```python
from build123d import *

# Parameters (mm, degrees)
SKETCH_1_W                         = 50
SKETCH_1_H                         = 50
SM_BASE_FLANGE_1_DEPTH             = 3
SM_EDGE_FLANGE_1_STRIP_W           = 13.4732
SM_EDGE_FLANGE_1_STRIP_H           = 3
SM_EDGE_FLANGE_1_STRIP_CUT_DEPTH   = 50
SM_EDGE_FLANGE_1_STRIP_2_W         = 13.4732
SM_EDGE_FLANGE_1_STRIP_2_H         = 3
SM_EDGE_FLANGE_1_STRIP_CUT_2_DEPTH = 50
SM_EDGE_FLANGE_1_DEPTH             = 50
SM_EDGE_FLANGE_1_BEND_DEPTH        = 50
SM_EDGE_FLANGE_2_STRIP_W           = 13.4732
SM_EDGE_FLANGE_2_STRIP_H           = 3
SM_EDGE_FLANGE_2_STRIP_CUT_DEPTH   = 50
SM_EDGE_FLANGE_2_STRIP_2_W         = 13.4732
SM_EDGE_FLANGE_2_STRIP_2_H         = 3
SM_EDGE_FLANGE_2_STRIP_CUT_2_DEPTH = 50
SM_EDGE_FLANGE_2_DEPTH             = 50
SM_EDGE_FLANGE_2_BEND_DEPTH        = 50
SKETCH_18_R                        = 6.5
CUT_EXTRUDE_1_DEPTH                = 98.103038058


# Sheet-metal steps are written as plain solids
with BuildPart() as part:
    # Sketch 1 → 基体-法兰1 (new body)
    with BuildSketch(Plane.XY):
        with Locations((25, 25)):
            Rectangle(SKETCH_1_W, SKETCH_1_H)
    extrude(amount=-SM_BASE_FLANGE_1_DEPTH)

    # 边线-法兰1 strip (across the edge) → 边线-法兰1 strip cut (cut)
    with BuildSketch(Plane(origin=(0, 50, -3), x_dir=(0, -1, 0), z_dir=(1, 0, 0))):
        with Locations((-6, -1.5)):
            Rectangle(SM_EDGE_FLANGE_1_STRIP_W, SM_EDGE_FLANGE_1_STRIP_H)
    extrude(amount=SM_EDGE_FLANGE_1_STRIP_CUT_DEPTH, mode=Mode.SUBTRACT)

    # 边线-法兰1 strip 2 (across the edge) → 边线-法兰1 strip cut 2 (cut)
    with BuildSketch(Plane(origin=(50, 0, -3), x_dir=(0, 1, 0), z_dir=(-1, 0, 0))):
        with Locations((-6, -1.5)):
            Rectangle(SM_EDGE_FLANGE_1_STRIP_2_W, SM_EDGE_FLANGE_1_STRIP_2_H)
    extrude(amount=SM_EDGE_FLANGE_1_STRIP_CUT_2_DEPTH, mode=Mode.SUBTRACT)

    # 边线-法兰1 section (across the edge) → 边线-法兰1 (add)
    with BuildSketch(Plane(origin=(0, 50, -3), x_dir=(0, -1, 0), z_dir=(1, 0, 0))):
        with BuildLine():
            Line((-3, 0.7366), (-3, 17))
            Line((-3, 17), (0, 17))
            Line((0, 17), (0, 0.7366))
            ThreePointArc((0, 0.7366), (0.215745145, 0.215745145), (0.7366, 0))
            Line((0.7366, 0), (0.7366, -3))
            ThreePointArc((0.7366, -3), (-1.905575199, -1.905575199), (-3, 0.7366))
        make_face()
    extrude(amount=SM_EDGE_FLANGE_1_DEPTH)

    # 边线-法兰1 section 2 (across the edge) → 边线-法兰1 bend (add)
    with BuildSketch(Plane(origin=(50, 0, -3), x_dir=(0, 1, 0), z_dir=(-1, 0, 0))):
        with BuildLine():
            Line((-3, 0.7366), (-3, 17))
            Line((-3, 17), (0, 17))
            Line((0, 17), (0, 0.7366))
            ThreePointArc((0, 0.7366), (0.215745145, 0.215745145), (0.7366, 0))
            Line((0.7366, 0), (0.7366, -3))
            ThreePointArc((0.7366, -3), (-1.905575199, -1.905575199), (-3, 0.7366))
        make_face()
    extrude(amount=SM_EDGE_FLANGE_1_BEND_DEPTH)

    # 边线-法兰2 strip (across the edge) → 边线-法兰2 strip cut (cut)
    with BuildSketch(Plane(origin=(0, -3, -20), x_dir=(0, 0, 1), z_dir=(1, 0, 0))):
        with Locations((-6, -1.5)):
            Rectangle(SM_EDGE_FLANGE_2_STRIP_W, SM_EDGE_FLANGE_2_STRIP_H)
    extrude(amount=SM_EDGE_FLANGE_2_STRIP_CUT_DEPTH, mode=Mode.SUBTRACT)

    # 边线-法兰2 strip 2 (across the edge) → 边线-法兰2 strip cut 2 (cut)
    with BuildSketch(Plane(origin=(50, 53, -20), x_dir=(0, 0, 1), z_dir=(-1, 0, 0))):
        with Locations((-6, -1.5)):
            Rectangle(SM_EDGE_FLANGE_2_STRIP_2_W, SM_EDGE_FLANGE_2_STRIP_2_H)
    extrude(amount=SM_EDGE_FLANGE_2_STRIP_CUT_2_DEPTH, mode=Mode.SUBTRACT)

    # 边线-法兰2 section (across the edge) → 边线-法兰2 (add)
    with BuildSketch(Plane(origin=(0, -3, -20), x_dir=(0, 0, 1), z_dir=(1, 0, 0))):
        with BuildLine():
            Line((-3, 0.7366), (-3, 27))
            Line((-3, 27), (0, 27))
            Line((0, 27), (0, 0.7366))
            ThreePointArc((0, 0.7366), (0.215745145, 0.215745145), (0.7366, 0))
            Line((0.7366, 0), (0.7366, -3))
            ThreePointArc((0.7366, -3), (-1.905575199, -1.905575199), (-3, 0.7366))
        make_face()
    extrude(amount=SM_EDGE_FLANGE_2_DEPTH)

    # 边线-法兰2 section 2 (across the edge) → 边线-法兰2 bend (add)
    with BuildSketch(Plane(origin=(50, 53, -20), x_dir=(0, 0, 1), z_dir=(-1, 0, 0))):
        with BuildLine():
            Line((-3, 0.7366), (-3, 27))
            Line((-3, 27), (0, 27))
            Line((0, 27), (0, 0.7366))
            ThreePointArc((0, 0.7366), (0.215745145, 0.215745145), (0.7366, 0))
            Line((0.7366, 0), (0.7366, -3))
            ThreePointArc((0.7366, -3), (-1.905575199, -1.905575199), (-3, 0.7366))
        make_face()
    extrude(amount=SM_EDGE_FLANGE_2_BEND_DEPTH)

    # 草图18 → 切除-拉伸1 (cut, through all)
    with BuildSketch(Plane.XY):
        with Locations((25, 25)):
            Circle(SKETCH_18_R)
    extrude(amount=-CUT_EXTRUDE_1_DEPTH, mode=Mode.SUBTRACT)


solid = part.part
```
Can you work these out from the model? Positions are in its coordinate system, mm. A direction names the side the tool comes from. Round coordinates to 2 decimals unless told otherwise and drop trailing zeros. Order: outer loops, then holes, each group sorted by start corner. A loop starts at its lowest first (then second) coordinate and runs counter-clockwise, first axis right, second up.
(1) On a 3-axis mill with a long thin cutter (end or side, diameter ignored), from which of +Z, -Z, +X, -X, +Y, -Y can I reach the whole of each face in a straight line? I mean faces 4 (the face through (25, 50, -12)), 5 (the face through (25, 53, -11)), 6 (the face through (25, -17, -20)). Say none if no direction works.
Results are:
face 4: -Z, +X, -X
face 5: +Z, +X, -X, +Y
face 6: +Z, +X, -X, -Y
(2) If we section it at D-D (x = 8): Please give me the cut outline in (y, z), plus the area to 3 significant figures.
Results are:
outline: (-30, -23) - (-3.74, -23) arc R3.74 ccw to (0, -19.26) - (0, -3.74) arc R0.74 cw to (0.74, -3) - (49.26, -3) arc R0.74 cw to (50, -3.74) - (50, -19.26) arc R3.74 ccw to (53.74, -23) - (80, -23) - (80, -20) - (53.74, -20) arc R0.74 cw to (53, -19.26) - (53, -3.74) arc R3.74 ccw to (49.26, 0) - (0.74, 0) arc R3.74 ccw to (-3, -3.74) - (-3, -19.26) arc R0.74 cw to (-3.74, -20) - (-30, -20) - close
area: 438 mm2
(3) We'd pull the mould along X, two halves only. Please class faces 1 (the face through (25, -17, -23)), 2 (the face through (0, 25, -2)), 3 (the face through (18.506, 25.286, -1.479)): +X half, -X half, draft (parallel to the pull), parting line (faces both ways), or undercut.
Results are:
face 1: draft
face 2: -X half
face 3: undercut
(4) If I drill on L1, parallel to Y at x = 9.5, z = -15.75; L2, parallel to Z at x = 13, y = 60; L3, parallel to Z at x = 44, y = 28, over which ranges is the centre line in solid material (lowest first)?
Results are:
L1: y = -3 to 0, 50 to 53
L2: z = -23 to -20
L3: z = -3 to 0
(5) If we section it at A-A (y = 25): Please give me the cut outline in (x, z), plus the area to 3 significant figures.
Results are:
outline: (0, -3) - (18.5, -3) - (18.5, 0) - (0, 0) - close; (31.5, -3) - (50, -3) - (50, 0) - (31.5, 0) - close
area: 111 mm2
(6) I'm going to push flat-ended pins straight in: pin 1 (8 mm diameter, centred on x = 29, z = -14, fed in from -Y); pin 2 (6 mm diameter, centred on x = 44.5, y = 62, fed in from +Z); pin 3 (8 mm diameter, centred on x = 13, z = -15, fed in from +Y). Where does each tip first touch, or does it pass through?
Results are:
pin 1: stops at y = -3
pin 2: stops at z = -20
pin 3: stops at y = 53
(7) If we section it at C-C (z = -13): Please give me the cut outline in (x, y), plus the area to 3 significant figures.
Results are:
outline: (0, -3) - (50, -3) - (50, 0) - (0, 0) - close; (0, 50) - (50, 50) - (50, 53) - (0, 53) - close
area: 300 mm2
(8) If we section it at B-B (x = 25): Please give me the cut outline in (y, z).
Results are:
outline: (-30, -23) - (-3.74, -23) arc R3.74 ccw to (0, -19.26) - (0, -3.74) arc R0.74 cw to (0.74, -3) - (18.5, -3) - (18.5, 0) - (0.74, 0) arc R3.74 ccw to (-3, -3.74) - (-3, -19.26) arc R0.74 cw to (-3.74, -20) - (-30, -20) - close; (31.5, -3) - (49.26, -3) arc R0.74 cw to (50, -3.74) - (50, -19.26) arc R3.74 ccw to (53.74, -23) - (80, -23) - (80, -20) - (53.74, -20) arc R0.74 cw to (53, -19.26) - (53, -3.74) arc R3.74 ccw to (49.26, 0) - (31.5, 0) - close
